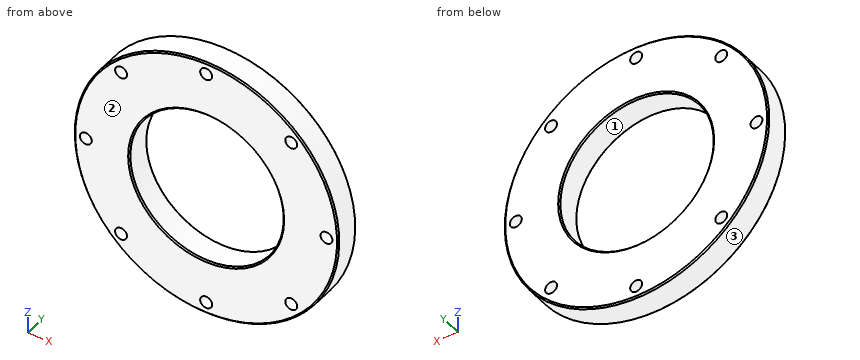
```python
from build123d import *

# Parameters (mm, degrees)
SKETCH1_R           = 50
SKETCH1_R_2         = 2.25
SKETCH1_R_3         = 29
BOSS_EXTRUDE1_DEPTH = 10
CHAMFER1_SIZE       = 0.5


with BuildPart() as part:
    # Sketch1 → Boss-Extrude1 (new body)
    with BuildSketch(Plane(origin=(0, 0, 0), x_dir=(1, 0, 0), z_dir=(0, 1, 0))):
        with Locations(Location((0, 0, 0), (0, 0, 270))):
            Circle(SKETCH1_R)
        with Locations(Location((0, 45.5, 0), (0, 0, 270))):
            Circle(SKETCH1_R_2, mode=Mode.SUBTRACT)
        with Locations(Location((32.173358544, 32.173358544, 0), (0, 0, 270))):
            Circle(SKETCH1_R_2, mode=Mode.SUBTRACT)
        with Locations(Location((45.5, 0, 0), (0, 0, 270))):
            Circle(SKETCH1_R_2, mode=Mode.SUBTRACT)
        with Locations(Location((32.173358544, -32.173358544, 0), (0, 0, 270))):
            Circle(SKETCH1_R_2, mode=Mode.SUBTRACT)
        with Locations(Location((0, -45.5, 0), (0, 0, 270))):
            Circle(SKETCH1_R_2, mode=Mode.SUBTRACT)
        with Locations(Location((-32.173358544, -32.173358544, 0), (0, 0, 270))):
            Circle(SKETCH1_R_2, mode=Mode.SUBTRACT)
        with Locations(Location((-45.5, 0, 0), (0, 0, 270))):
            Circle(SKETCH1_R_2, mode=Mode.SUBTRACT)
        with Locations(Location((-32.173358544, 32.173358544, 0), (0, 0, 270))):
            Circle(SKETCH1_R_2, mode=Mode.SUBTRACT)
        with Locations(Location((0, 0, 0), (0, 0, 270))):
            Circle(SKETCH1_R_3, mode=Mode.SUBTRACT)
    extrude(amount=BOSS_EXTRUDE1_DEPTH)

    # Chamfer1
    chamfer1_edges = [part.edges().sort_by_distance(p)[0] for p in [
        (0, 0, -50),
        (0, 10, -50),
        (0, 0, -29),
        (0, 10, -29),
    ]]
    chamfer(chamfer1_edges, length=CHAMFER1_SIZE)


solid = part.part
```
Build history of the part. All positions in model axes, mm. Face numbers are marked on the shaded views. Give positions to 0.01 mm unless a question says otherwise; leave off trailing zeros. Order: outer loops, then holes, each group sorted by start corner. A loop starts at its lowest first (then second) coordinate and runs counter-clockwise, first axis right, second up. Notation, with made-up numbers: M -23,78 L 5,78 A25 ccw 5,108 Z; hole C 29,29 d11. An arc over 180 degrees is marked long. Return JSON: item names as keys, results as strings.
Q1. Flat gauge pins, fed straight in: pin 1 (5 mm diameter, centred on y = 2.5, z = 37, fed in from +X); pin 2 (6 mm diameter, centred on x = -30, y = 7, fed in from +Z); pin 3 (2 mm diameter, centred on y = 2.5, z = -30.5, fed in from +X). Where does each tip first touch, or does it go through?
Answer list:
{"pin 1": "stops at x = 36.19", "pin 2": "stops at z = 42.08", "pin 3": "stops at x = 40.37"}
Q2. Band-saw the part on B-B (y = 7.5). Count the separate pieces of the cut face and the enclosed holes in it, then the cut area to 3 significant figures.
Answer list:
{"separate pieces": "1", "enclosed holes": "9", "area": "5,080 mm^2"}
Q3. Wall check: probe 1 along X at (y, z) = (3.5, 0); probe 2 along X at (y, z) = (4.5, 33.5); probe 3 along X at (y, z) = (2.5, -34). Give the ranges that are in metal, low to high. Write a range as from..to.
Answer list:
{"probe 1": "x = -50..-47.75, -43.25..-29, 29..43.25, 47.75..50", "probe 2": "x = -37.12..-33.99, -30.36..30.36, 33.99..37.12", "probe 3": "x = -36.66..-33.49, -30.86..30.86, 33.49..36.66"}
Q4. Two-plate mould, pull along Z, no slides. Class the marked faces 1, 2 and 3: pulls with the +Z half, pulls with the -Z half, needs draft (parallel to the pull), parting line crosses it, or undercut.
Answer list:
{"face 1": "undercut", "face 2": "needs draft", "face 3": "parting line crosses it"}
Q5. Band-saw the part on A-A (z = 0). Give the cut face in (x, y), then the cut area to 3 significant figures.
Answer list:
{"outline": "M -50,0.5 L -49.5,0 L -47.75,0 L -47.75,10 L -49.5,10 L -50,9.5 Z; M -43.25,0 L -29.5,0 L -29,0.5 L -29,9.5 L -29.5,10 L -43.25,10 Z; M 29,0.5 L 29.5,0 L 43.25,0 L 43.25,10 L 29.5,10 L 29,9.5 Z; M 47.75,0 L 49.5,0 L 50,0.5 L 50,9.5 L 49.5,10 L 47.75,10 Z", "area": "329 mm^2"}
